Can you work these out from the model? Positions are in its coordinate system, mm. Give positions to 0.01 mm unless a question says otherwise; leave off trailing zeros. Loops run counter-clockwise (first coordinate to the right, second up) from the corner with the lowest first, then second, coordinate; pieces in that order, holes last. Notation, with made-up numbers: (-32, 69) -> (1, 69) arc R22 cw to (1, 108) -> close; hole circle Ø7 at (65.5, 50). An arc over 180 degrees is marked (long way). Use CSV: the item, a comma, the result in double quotes.
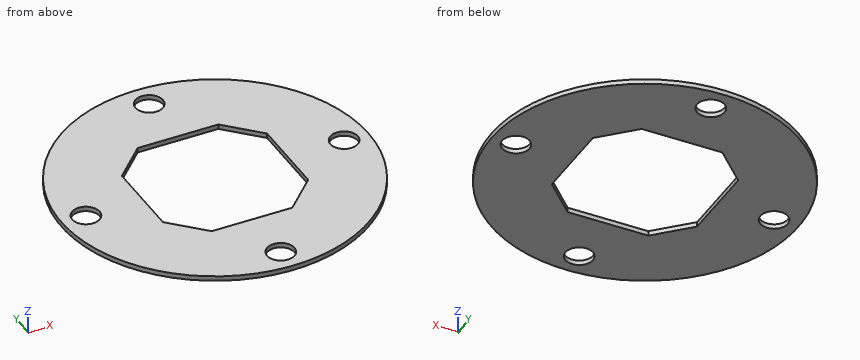
Autodesk Inventor part; units mm, degrees
ref_plane "YZ Plane" through (0, 0, 0) normal (1, 0, 0) x (0, 1, 0)
ref_plane "XZ Plane" through (0, 0, 0) normal (0, 1, 0) x (-1, 0, 0)
ref_plane "XY Plane" through (0, 0, 0) normal (0, 0, 1) x (1, 0, 0)
sketch "Sketch1" plane through (0, 0, 0) normal (0, 0, 1) x (1, 0, 0)
  circle A0 centre (0, 0) radius 95
  line L0 (45, 45) -> (-45, 45)
  line L1 (-45, 45) -> (-45, -45)
  line L2 (-45, -45) -> (45, -45)
  line L3 (45, -45) -> (45, 45)
  line L4 (45, 45) -> (-45, -45) construction
  line L5 (-45, 45) -> (45, -45) construction
  dimension "d157" = 190
  dimension "d158" = 90
  dimension "d159" = 90
extrude "Plate5" add sketch "Sketch1" along normal blind 3
sketch "Sketch7" plane through (0, 0, 0) normal (0, 0, -1) x (-1, 0, 0)
  circle A0 centre (0, 80) radius 8.5
  point P0 (0, 0)
  dimension "d160" = 17
  dimension "d161" = 80
extrude "Cut1" cut sketch "Sketch7" against normal blind 3
pattern_circular "Circular Pattern1" count 4 over 360 about axis through (0, 0, -10) along (0, 0, 1) of "Cut1"
chamfer "Corner Chamfer2" distance 20 angle 45 4 edges at (-45, -45, 1.5) (45, -45, 1.5) (-45, 45, 1.5) (45, 45, 1.5)
properties part number "PNS 1651 FDS MAIN  FLANGE" material "Stainless Steel"
(1) If we section it at C-C, the plane z = 1.35: Write out the boundary of the cut face in (x, y), then the cut area to 3 significant figures.
Answer sheet:
outline,"circle Ø190 at (0, 0); hole circle Ø17 at (-80, 0); hole (-45, -25) -> (-25, -45) -> (25, -45) -> (45, -25) -> (45, 25) -> (25, 45) -> (-25, 45) -> (-45, 25) -> close; hole circle Ø17 at (0, -80); hole circle Ø17 at (0, 80); hole circle Ø17 at (80, 0)"
area,"20,100 mm2"
(2) If I drill on L1, parallel to Y at x = 0, z = 0.8; L2, parallel to X at y = 5.5, z = 2; L3, parallel to Y at x = -4, z = 2.05, over which ranges is the centre line in solid material (lowest first)? Write a range as from..to.
Answer sheet:
L1,"y = -95..-88.5, -71.5..-45, 45..71.5, 88.5..95"
L2,"x = -94.84..-86.48, -73.52..-45, 45..73.52, 86.48..94.84"
L3,"y = -94.92..-87.5, -72.5..-45, 45..72.5, 87.5..94.92"
(3) If we section it at D-D, the plane y = -80: Write out the boundary of the cut face in (x, z), then the cut area to 3 significant figures.
Answer sheet:
outline,"(-51.23, 0) -> (-8.5, 0) -> (-8.5, 3) -> (-51.23, 3) -> close; (8.5, 0) -> (51.23, 0) -> (51.23, 3) -> (8.5, 3) -> close"
area,"256 mm2"
(4) If we section it at B-B, the plane x = 14.5: Write out the boundary of the cut face in (y, z), then the cut area to 3 significant figures.
Answer sheet:
outline,"(-93.89, 0) -> (-45, 0) -> (-45, 3) -> (-93.89, 3) -> close; (45, 0) -> (93.89, 0) -> (93.89, 3) -> (45, 3) -> close"
area,"293 mm2"
(5) If we section it at A-A, the plane y = 0: Write out the boundary of the cut face in (x, z), then the cut area to 3 significant figures.
Answer sheet:
outline,"(-95, 0) -> (-88.5, 0) -> (-88.5, 3) -> (-95, 3) -> close; (-71.5, 0) -> (-45, 0) -> (-45, 3) -> (-71.5, 3) -> close; (45, 0) -> (71.5, 0) -> (71.5, 3) -> (45, 3) -> close; (88.5, 0) -> (95, 0) -> (95, 3) -> (88.5, 3) -> close"
area,"198 mm2"
(6) Will these pins go through, and if not, where does the flat tip stop? pin 1 Ø8 at (x, y) = (64.5, -70) entering from +Z; pin 2 Ø13.5 at (x, y) = (0, -80) entering from +Z; pin 3 Ø0.9 at (x, z) = (4.5, 1.5) entering from +Y.
Answer sheet:
pin 1,"stops at z = 3"
pin 2,"passes through"
pin 3,"stops at y = 94.91"
